Part model, mm, in its own coordinate system. Face numbers are marked on the shaded views. A direction names the side the tool comes from. Round coordinates to 2 decimals unless told otherwise and drop trailing zeros.
(1) Cut at A-A on x = 5.5. Count the separate pieces of the cut face and the enclosed holes in it, then the cut area to 3 significant figures.
(2) Probe probe 1 along Y at (x, z) = (0, -21.25); probe 2 along X at (y, z) = (-9, -3.5); probe 3 along Y at (x, z) = (20.5, -17.5). List the from-to ranges inside material, lowest first.
(3) Mould opens along X. For the marked faces 5, 6 and 7 say: +X half, -X half, draft (parallel to the pull), parting line (faces both ways), or undercut.
(4) Flat gauge pins, fed straight in: pin 1 (0.6 mm diameter, centred on x = -4, y = -24, fed in from +Z); pin 2 (2 mm diameter, centred on x = -7.5, z = -24.5, fed in from -Y); pin 3 (0.6 mm diameter, centred on y = 24, z = -5, fed in from -X). Where does each tip first touch, or does it go through?
(5) Tool access for the marked faces 1, 2, 3 and 4: list every direction of +Z, -Z, +X, -X, +Y, -Y with a clear straight run to the whole face (end or side of a thin tool).
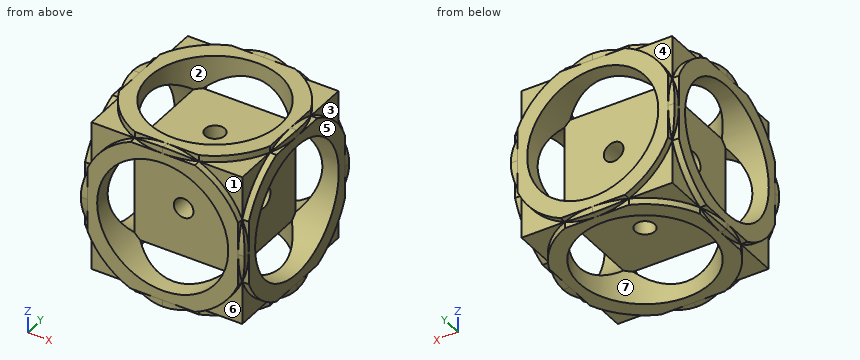
from build123d import *

# Parameters (mm, degrees)
F0_W          = 50
F0_H          = 50
F1_DEPTH      = 25
F1_DEPTH_BACK = 25
F3_D          = 40
F5_D          = 40
F7_D          = 40
F8_W          = 30
F8_H          = 30
F9_DEPTH      = 15
F9_DEPTH_BACK = 15
F17_DEPTH     = 2
F18_DEPTH     = 2
F19_DEPTH     = 2
F20_DEPTH     = 2
F21_DEPTH     = 2
F22_DEPTH     = 2
F23_DEPTH     = 2
F25_D         = 6
F27_D         = 6
F29_D         = 6


with BuildPart() as f1:
    # F0 (on Front) → F1 (new body, two sides)
    with BuildSketch(Plane.XZ) as f1_sk:
        Rectangle(F0_W, F0_H)
    extrude(amount=F1_DEPTH)
    extrude(f1_sk.sketch, amount=-F1_DEPTH_BACK)

    # F3 (through all)
    with Locations(Plane.YZ.offset(25)):
        with Locations((0, 0)):
            Hole(F3_D / 2)

    # F5 (through all)
    with Locations(Plane.XY.offset(25)):
        with Locations((0, 0)):
            Hole(F5_D / 2)

    # F7 (through all)
    with Locations(Plane.XZ.offset(25)):
        with Locations((0, 0)):
            Hole(F7_D / 2)

    # F8 (on Top) → F9 (join, two sides)
    with BuildSketch(Plane.XY) as f9_sk:
        Rectangle(F8_W, F8_H)
    extrude(amount=F9_DEPTH)
    extrude(f9_sk.sketch, amount=-F9_DEPTH_BACK)

    # F10 (on face) → F17 (cut)
    with BuildSketch(Plane(origin=(0, 25, 0), x_dir=(-1, 0, 0), z_dir=(0, 1, 0))):
        with BuildLine():
            ThreePointArc((0, 25), (17.6776695297, 17.6776695297), (25, 0))
            Line((25, 0), (25, 25))
            Line((25, 25), (0, 25))
        make_face()
        with BuildLine():
            ThreePointArc((-25, 2.61e-08), (-17.6776695204, 17.6776695389), (0, 25))
            Line((0, 25), (-25, 25))
            Line((-25, 25), (-25, 2.61e-08))
        make_face()
        with BuildLine():
            Line((-25, -25), (-5.83e-08, -25))
            ThreePointArc((-5.83e-08, -25), (-17.6776695595, -17.6776694998), (-25, 2.61e-08))
            Line((-25, 2.61e-08), (-25, -25))
        make_face()
        with BuildLine():
            Line((25, -25), (25, 0))
            ThreePointArc((25, 0), (17.677669509, -17.6776695503), (-5.83e-08, -25))
            Line((-5.83e-08, -25), (25, -25))
        make_face()
    extrude(amount=F17_DEPTH, mode=Mode.SUBTRACT)

    # F15 (on face) → F18 (cut)
    with BuildSketch(Plane.XZ.offset(25)):
        with BuildLine():
            ThreePointArc((-25, 2.61e-08), (-17.6776695204, 17.6776695389), (0, 25))
            Line((0, 25), (-25, 25))
            Line((-25, 25), (-25, 2.61e-08))
        make_face()
        with BuildLine():
            Line((-25, -25), (-5.83e-08, -25))
            ThreePointArc((-5.83e-08, -25), (-17.6776695595, -17.6776694998), (-25, 2.61e-08))
            Line((-25, 2.61e-08), (-25, -25))
        make_face()
        with BuildLine():
            Line((25, -25), (25, 0))
            ThreePointArc((25, 0), (17.677669509, -17.6776695503), (-5.83e-08, -25))
            Line((-5.83e-08, -25), (25, -25))
        make_face()
        with BuildLine():
            ThreePointArc((0, 25), (17.6776695297, 17.6776695297), (25, 0))
            Line((25, 0), (25, 25))
            Line((25, 25), (0, 25))
        make_face()
    extrude(amount=-F18_DEPTH, mode=Mode.SUBTRACT)

    # F12 (on face) → F19 (cut)
    with BuildSketch(Plane.XY.offset(25)):
        with BuildLine():
            Line((-25, -25), (-5.83e-08, -25))
            ThreePointArc((-5.83e-08, -25), (-17.6776695595, -17.6776694998), (-25, 2.61e-08))
            Line((-25, 2.61e-08), (-25, -25))
        make_face()
        with BuildLine():
            ThreePointArc((-25, 2.61e-08), (-17.6776695204, 17.6776695389), (0, 25))
            Line((0, 25), (-25, 25))
            Line((-25, 25), (-25, 2.61e-08))
        make_face()
        with BuildLine():
            ThreePointArc((0, 25), (17.6776695297, 17.6776695297), (25, 0))
            Line((25, 0), (25, 25))
            Line((25, 25), (0, 25))
        make_face()
        with BuildLine():
            Line((25, -25), (25, 0))
            ThreePointArc((25, 0), (17.677669509, -17.6776695503), (-5.83e-08, -25))
            Line((-5.83e-08, -25), (25, -25))
        make_face()
    extrude(amount=-F19_DEPTH, mode=Mode.SUBTRACT)

    # F13 (on face) → F20 (cut)
    with BuildSketch(Plane.YZ.offset(25)):
        with BuildLine():
            ThreePointArc((-25, 2.61e-08), (-17.6776695204, 17.6776695389), (0, 25))
            Line((0, 25), (-25, 25))
            Line((-25, 25), (-25, 2.61e-08))
        make_face()
        with BuildLine():
            ThreePointArc((0, 25), (17.6776695297, 17.6776695297), (25, 0))
            Line((25, 0), (25, 25))
            Line((25, 25), (0, 25))
        make_face()
        with BuildLine():
            Line((25, -25), (25, 0))
            ThreePointArc((25, 0), (17.677669509, -17.6776695503), (-5.83e-08, -25))
            Line((-5.83e-08, -25), (25, -25))
        make_face()
        with BuildLine():
            Line((-25, -25), (-5.83e-08, -25))
            ThreePointArc((-5.83e-08, -25), (-17.6776695595, -17.6776694998), (-25, 2.61e-08))
            Line((-25, 2.61e-08), (-25, -25))
        make_face()
    extrude(amount=-F20_DEPTH, mode=Mode.SUBTRACT)

    # F16 (on face) → F21 (cut)
    with BuildSketch(Plane(origin=(0, 25, 0), x_dir=(-1, 0, 0), z_dir=(0, 1, 0))):
        with BuildLine():
            ThreePointArc((-25, 2.61e-08), (-17.6776695204, 17.6776695389), (0, 25))
            Line((0, 25), (-25, 25))
            Line((-25, 25), (-25, 2.61e-08))
        make_face()
        with BuildLine():
            ThreePointArc((0, 25), (17.6776695297, 17.6776695297), (25, 0))
            Line((25, 0), (25, 25))
            Line((25, 25), (0, 25))
        make_face()
        with BuildLine():
            Line((25, -25), (25, 0))
            ThreePointArc((25, 0), (17.677669509, -17.6776695503), (-5.83e-08, -25))
            Line((-5.83e-08, -25), (25, -25))
        make_face()
        with BuildLine():
            Line((-25, -25), (-5.83e-08, -25))
            ThreePointArc((-5.83e-08, -25), (-17.6776695595, -17.6776694998), (-25, 2.61e-08))
            Line((-25, 2.61e-08), (-25, -25))
        make_face()
    extrude(amount=-F21_DEPTH, mode=Mode.SUBTRACT)

    # F11 (on face) → F22 (cut)
    with BuildSketch(Plane(origin=(-25, 0, 0), x_dir=(0, -1, 0), z_dir=(-1, 0, 0))):
        with BuildLine():
            ThreePointArc((-25, 2.61e-08), (-17.6776695204, 17.6776695389), (0, 25))
            Line((0, 25), (-25, 25))
            Line((-25, 25), (-25, 2.61e-08))
        make_face()
        with BuildLine():
            ThreePointArc((0, 25), (17.6776695297, 17.6776695297), (25, 0))
            Line((25, 0), (25, 25))
            Line((25, 25), (0, 25))
        make_face()
        with BuildLine():
            Line((25, -25), (25, 0))
            ThreePointArc((25, 0), (17.677669509, -17.6776695503), (-5.83e-08, -25))
            Line((-5.83e-08, -25), (25, -25))
        make_face()
        with BuildLine():
            Line((-25, -25), (-5.83e-08, -25))
            ThreePointArc((-5.83e-08, -25), (-17.6776695595, -17.6776694998), (-25, 2.61e-08))
            Line((-25, 2.61e-08), (-25, -25))
        make_face()
    extrude(amount=-F22_DEPTH, mode=Mode.SUBTRACT)

    # F14 (on face) → F23 (cut)
    with BuildSketch(Plane(origin=(0, 0, -25), x_dir=(1, 0, 0), z_dir=(0, 0, -1))):
        with BuildLine():
            ThreePointArc((-25, 2.61e-08), (-17.6776695204, 17.6776695389), (0, 25))
            Line((0, 25), (-25, 25))
            Line((-25, 25), (-25, 2.61e-08))
        make_face()
        with BuildLine():
            Line((-25, -25), (-5.83e-08, -25))
            ThreePointArc((-5.83e-08, -25), (-17.6776695595, -17.6776694998), (-25, 2.61e-08))
            Line((-25, 2.61e-08), (-25, -25))
        make_face()
        with BuildLine():
            Line((25, -25), (25, 0))
            ThreePointArc((25, 0), (17.677669509, -17.6776695503), (-5.83e-08, -25))
            Line((-5.83e-08, -25), (25, -25))
        make_face()
        with BuildLine():
            ThreePointArc((0, 25), (17.6776695297, 17.6776695297), (25, 0))
            Line((25, 0), (25, 25))
            Line((25, 25), (0, 25))
        make_face()
    extrude(amount=-F23_DEPTH, mode=Mode.SUBTRACT)

    # F25 (through all)
    with Locations(Plane.YZ.offset(15)):
        with Locations((0, 0)):
            Hole(F25_D / 2)

    # F27 (through all)
    with Locations(Plane(origin=(0, 15, 0), x_dir=(-1, 0, 0), z_dir=(0, 1, 0))):
        with Locations((0, 0)):
            Hole(F27_D / 2)

    # F29 (through all)
    with Locations(Plane(origin=(0, 0, -15), x_dir=(1, 0, 0), z_dir=(0, 0, -1))):
        with Locations((0, 0)):
            Hole(F29_D / 2)


solid = f1.part
Final values:
1. separate pieces: 5
1. enclosed holes: 1
1. area: 997 mm2
2. probe 1: y = -25 to -20, 20 to 25
2. probe 2: x = -15 to 15
2. probe 3: y = -23 to -9.68, 9.68 to 23
3. face 5: +X half
3. face 6: draft
3. face 7: undercut
4. pin 1: stops at z = 24.72
4. pin 2: stops at y = -24.12
4. pin 3: stops at x = -24.55
5. face 1: +Z, +X, -Y
5. face 2: +Z
5. face 3: +Z, +X, +Y
5. face 4: +Z, -X, +Y
